Design review of the part shown in the three views and the two pictorial views. Dimensions are in mm from the part's minimum x, y and z. Round coordinates to 2 decimals unless told otherwise and drop trailing zeros. Order: outer loops, then holes, each group sorted by start corner. A loop starts at its lowest first (then second) coordinate and runs counter-clockwise, first axis right, second up.
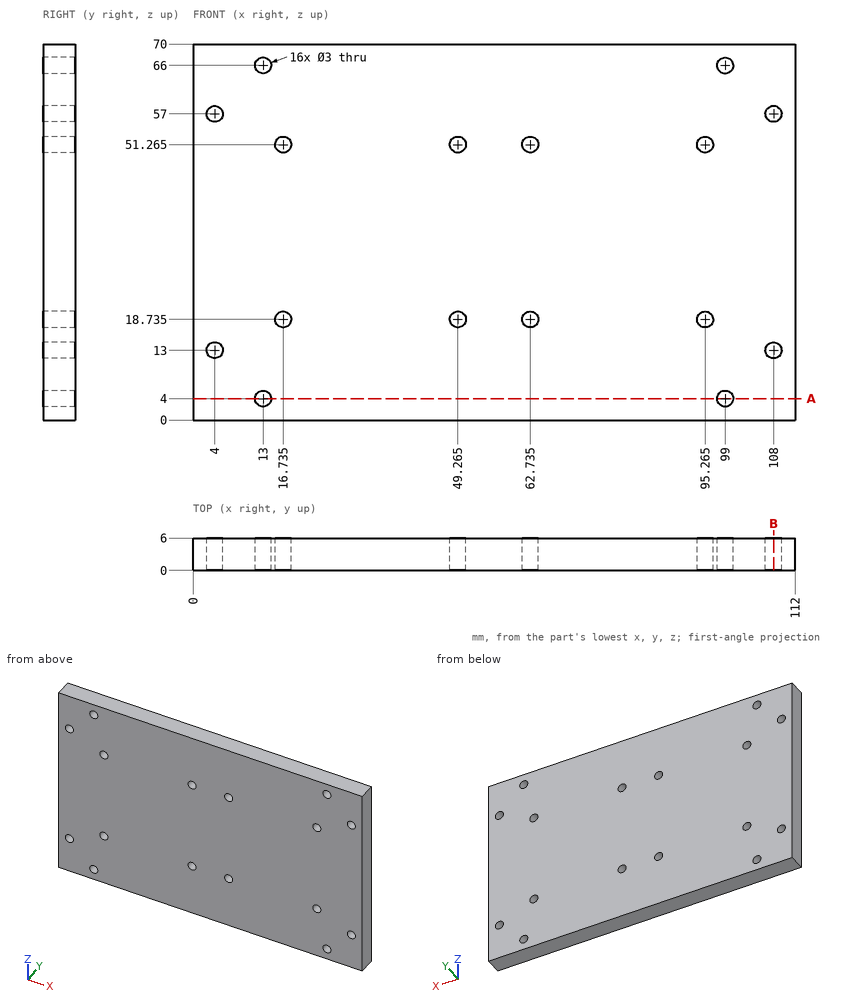
(1) Add section B-B on x = 108. Give the boundary of the cut face in (y, z).
(2) Add section A-A on z = 4. Give the boundary of the cut face in (x, y).
(3) Wall thickness on L1, parallel to Z at x = 108, y = 3.4; L2, parallel to Z at x = 99, y = 3.85; L3, parallel to X at y = 4.7, z = 12.5: over which ranges is each line inside the solid? List them lowest first.
Here are the results:
1. outline: (0, 0) - (6, 0) - (6, 11.5) - (0, 11.5) - close; (0, 14.5) - (6, 14.5) - (6, 55.5) - (0, 55.5) - close; (0, 58.5) - (6, 58.5) - (6, 70) - (0, 70) - close
2. outline: (0, 0) - (11.5, 0) - (11.5, 6) - (0, 6) - close; (14.5, 0) - (97.5, 0) - (97.5, 6) - (14.5, 6) - close; (100.5, 0) - (112, 0) - (112, 6) - (100.5, 6) - close
3. L1: z = 0 to 11.5, 14.5 to 55.5, 58.5 to 70
3. L2: z = 0 to 2.5, 5.5 to 64.5, 67.5 to 70
3. L3: x = 0 to 2.59, 5.41 to 106.59, 109.41 to 112
